Here's how the part is built. I have some questions about the finished solid (model axes, mm). Round coordinates to 2 decimals unless told otherwise and drop trailing zeros. Order: outer loops, then holes, each group sorted by start corner. A loop starts at its lowest first (then second) coordinate and runs counter-clockwise, first axis right, second up.
```python
from build123d import *

# Parameters (mm, degrees)
SKETCH_1_W        = 230
SKETCH_1_H        = 70
SKETCH_1_R        = 13
EXTRUDE_365_DEPTH = 16
CHAMFER_1_SIZE    = 2


with BuildPart() as part:
    # 草图1 → Extrude 365 (new body)
    with BuildSketch(Plane.XY):
        Rectangle(SKETCH_1_W, SKETCH_1_H)
        Circle(SKETCH_1_R, mode=Mode.SUBTRACT)
        with Locations((80, 0)):
            Circle(SKETCH_1_R, mode=Mode.SUBTRACT)
        with Locations((-80, 0)):
            Circle(SKETCH_1_R, mode=Mode.SUBTRACT)
    extrude(amount=EXTRUDE_365_DEPTH)

    # 倒角1
    chamfer_1_edges = [part.edges().sort_by_distance(p)[0] for p in [
        (115, 0, 16),
        (-13, 0, 0),
        (-13, 0, 16),
        (0, 35, 16),
        (67, 0, 0),
        (67, 0, 16),
        (-93, 0, 0),
        (-93, 0, 16),
        (-115, 0, 16),
        (0, 35, 0),
        (115, 0, 0),
        (0, -35, 0),
        (-115, 0, 0),
        (0, -35, 16),
    ]]
    chamfer(chamfer_1_edges, length=CHAMFER_1_SIZE)


solid = part.part
```
1. If we section it at A-A, the plane z = 7: Write out the boundary of the cut face in (x, y).
Evaluation:
outline: (-115, -35) - (115, -35) - (115, 35) - (-115, 35) - close; hole circle Ø26 at (-80, 0); hole circle Ø26 at (0, 0); hole circle Ø26 at (80, 0)
2. If we section it at B-B, the plane x = -80: Write out the boundary of the cut face in (y, z).
Evaluation:
outline: (-35, 2) - (-33, 0) - (-15, 0) - (-13, 2) - (-13, 14) - (-15, 16) - (-33, 16) - (-35, 14) - close; (13, 2) - (15, 0) - (33, 0) - (35, 2) - (35, 14) - (33, 16) - (15, 16) - (13, 14) - close
3. If we section it at C-C, the plane y = 0: State how many separate pieces and enclosed holes the cut face has, and give its area (3 significant figures).
Evaluation:
separate pieces: 4
enclosed holes: 0
area: 2,400 mm2
4. I need wall thicknesses on probe 1 along Y at (x, z) = (-80, 4.5); probe 2 along X at (y, z) = (-9, 12.5); probe 3 along X at (y, z) = (-4, 8.75). Which ranges of each line are inside material? Lowest first, please.
Evaluation:
probe 1: y = -35 to -13, 13 to 35
probe 2: x = -115 to -89.38, -70.62 to -9.38, 9.38 to 70.62, 89.38 to 115
probe 3: x = -115 to -92.37, -67.63 to -12.37, 12.37 to 67.63, 92.37 to 115
5. If we mould it in two halves opening along Y, with no side actions, what happens to faces 1 (the flat face through (-2, 35, 8)), 2 (the conical face through (12.519, 3.942, 14.125)), 3 (the flat face through (-2, -35, 8)), 4 (the cylindrical face through (67.013, 0.572, 7.916))? For each: released by +Y, released by -Y, zero draft, split by the parting line, or undercut.
Evaluation:
face 1: released by +Y
face 2: undercut
face 3: released by -Y
face 4: undercut
